For this review, take the finished solid that the model builds, in its own axes (mm). A direction names the side the tool comes from. Give positions to 0.01 mm unless a question says otherwise; leave off trailing zeros. Loops run counter-clockwise (first coordinate to the right, second up) from the corner with the lowest first, then second, coordinate; pieces in that order, holes last. Notation, with made-up numbers: (36, -8.5) - (56, -8.5) arc R25 ccw to (56, 6.5) - close; hole circle Ø1 at (9.25, -23.5). An arc over 180 degrees is marked (long way). Use CSV: the item, a comma, the result in double quotes. Start each with the question number.
1. Wall thickness on line 1 (Y direction, x = 4, z = 11.5); line 2 (X direction, y = -17.5, z = 12); line 3 (Y direction, x = 5.75, z = 9.25): over which ranges is each line inside the solid? List them lowest first.
2. Mouldability with a two-part tool opening along X and no side actions: class faces 4 (the flat face through (5, -12, 17.462)), 5 (the flat face through (-6.2, -5.2, 8.6)), 6 (the flat face through (18, -15.147, 9)) as pulls with the +X half, pulls with the -X half, needs draft (parallel to the pull), parting line crosses it, or undercut.
3. Take a section at B-B on x = 18.5. Give the boundary of the cut face in (y, z).
4. Take a section at C-C on y = -17.5. Give the boundary of the cut face in (x, z), plus the area to 3 significant figures.
5. For pin 1 (2 mm diameter, centred on y = -16, z = 6, fed in from -X); pin 2 (3 mm diameter, centred on x = -2, z = 8, fed in from -Y); pin 3 (1 mm diameter, centred on x = 11, z = 13, fed in from -Y); pin 4 (2 mm diameter, centred on x = 6.5, y = -9, fed in from +Z), all flat-tipped, find the tip position at first contact; note any pin that passes through.
6. For faces 1 (the flat face through (19.276, -14, 9)), 2 (the flat face through (19, -12.369, 9)), 3 (the flat face through (17.462, -13, 9)), list the 3-axis set-ups (+Z, -Z, +X, -X, +Y, -Y) from which the entire face can be reached by the end or side of a thin tool; tool diameter is ignored.
7. Take a section at D-D on x = 6. Give the boundary of the cut face in (y, z).
```python
from build123d import *

# Parameters (mm, degrees)
BOSS_EXTRUDE1_DEPTH = 17.4625


with BuildPart() as part:
    # Sketch1 → Boss-Extrude1 (new body)
    with BuildSketch(Plane.XY):
        with BuildLine():
            Line((17.165632348, -15.146713758), (19.25021974, -15.146713758))
            ThreePointArc((19.25021974, -15.146713758), (19.268180252, -15.139274271), (19.27561974, -15.121313758))
            Line((19.27561974, -15.121313758), (19.27561974, -13.771938758))
            Line((19.27561974, -13.771938758), (17.462436286, -13.771938758))
            Line((17.462436286, -13.771938758), (17.462436286, -12.368588758))
            Line((17.462436286, -12.368588758), (20.535179361, -12.368588758))
            ThreePointArc((20.535179361, -12.368588758), (21.54921714, -16.988767417), (17.921869262, -20.024664455))
            ThreePointArc((17.921869262, -20.024664455), (6.385080471, -18.490906221), (-3.456137762, -12.277989546))
            ThreePointArc((-3.456137762, -12.277989546), (-4.173487151, -11.127601987), (-4.620530274, -9.847705847))
            Line((-4.620530274, -9.847705847), (-7.811999534, -0.450394448))
            Line((-7.811999534, -0.450394448), (-0.904044887, 1.896214799))
            Line((-0.904044887, 1.896214799), (2.118621316, -7.011726883))
            ThreePointArc((2.118621316, -7.011726883), (3.222227995, -8.118323003), (3.87016333, -9.540533423))
            ThreePointArc((3.87016333, -9.540533423), (4.239027768, -10.27403939), (4.736122073, -10.927483519))
            ThreePointArc((4.736122073, -10.927483519), (4.769468956, -11.008731963), (4.742121249, -11.092191097))
            Line((4.742121249, -11.092191097), (4.651650579, -11.206452905))
            ThreePointArc((4.651650579, -11.206452905), (4.626334833, -11.308376501), (4.686416978, -11.394512685))
            ThreePointArc((4.686416978, -11.394512685), (6.198075477, -12.211534349), (7.770150037, -12.905232694))
            ThreePointArc((7.770150037, -12.905232694), (7.952657914, -13.051135413), (8.021441195, -13.274441457))
            Line((8.021441195, -13.274441457), (8.021441195, -13.569821942))
            ThreePointArc((8.021441195, -13.569821942), (8.094604206, -13.799430989), (8.287118368, -13.944384215))
            ThreePointArc((8.287118368, -13.944384215), (12.665355124, -14.99614841), (17.165632348, -15.146713758))
        make_face()
    extrude(amount=BOSS_EXTRUDE1_DEPTH)


solid = part.part
```
Check result:
1,line 1,"y = -17.5 to -9.84"
1,line 2,"x = 4.01 to 21.34"
1,line 3,"y = -18.25 to -11.99"
2,face 4,"needs draft"
2,face 5,"pulls with the -X half"
2,face 6,"undercut"
3,outline,"(-19.9, 0) - (-15.15, 0) - (-15.15, 17.46) - (-19.9, 17.46) - close; (-13.77, 0) - (-12.37, 0) - (-12.37, 17.46) - (-13.77, 17.46) - close"
4,outline,"(4.01, 0) - (21.34, 0) - (21.34, 17.46) - (4.01, 17.46) - close"
4,area,"303 mm²"
5,pin 1,"stops at x = -0.23"
5,pin 2,"stops at y = -14.8"
5,pin 3,"stops at y = -19.8"
5,pin 4,"passes through"
6,face 1,"+Z, -Z"
6,face 2,"+Z, -Z, +X, +Y"
6,face 3,"+Z, -Z, +Y"
7,outline,"(-18.35, 0) - (-12.11, 0) - (-12.11, 17.46) - (-18.35, 17.46) - close"
